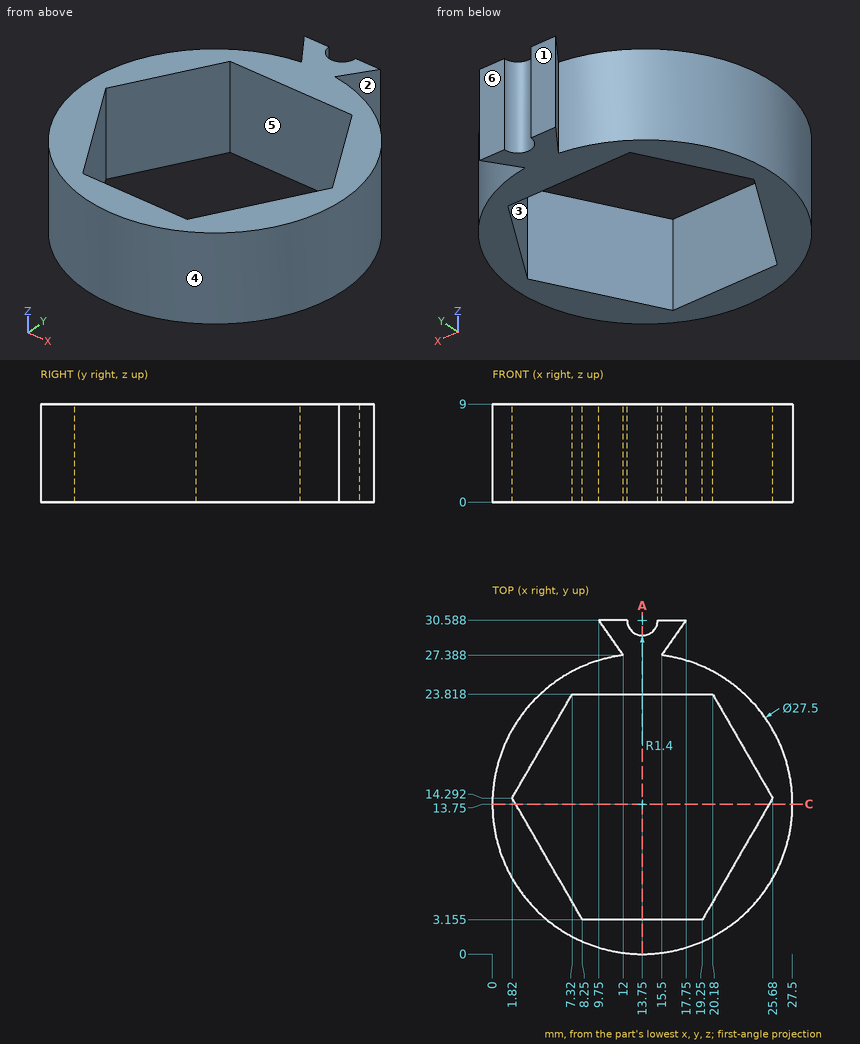
Source: three-view drawing plus pictorial views. Frame: mm from the lowest corner of the part. A direction names the side the tool comes from. Round coordinates to 2 decimals unless told otherwise and drop trailing zeros. Loops run counter-clockwise (first coordinate to the right, second up) from the corner with the lowest first, then second, coordinate; pieces in that order, holes last. Notation, with made-up numbers: (19, 38.5) - (63, 38.5) arc R27 ccw to (63, 57.5) - close; hole circle Ø6 at (45, -32.75). An arc over 180 degrees is marked (long way). Write item = value, one per line. Start each with the question number.
Item 1: First-contact query: pin 1 Ø1 at (x, z) = (11.5, 3.5) entering from -Y; pin 2 Ø5 at (y, z) = (21.5, 2) entering from -X; pin 3 Ø1 at (x, z) = (19, 3) entering from +Y; pin 4 Ø1.5 at (x, y) = (6, 9) entering from -Z. Flat tips, straight axial feed; report the tip coordinate or a pass-through.
Item 2: Section query C-C on y = 13.75. Output: boundary loops of the cut face in (x, z), plus the area to 3 significant figures.
Item 3: Reachability of the marked faces 1, 2 and 3 from +Z, -Z, +X, -X, +Y, -Y: full face, straight path, thin tool, end or side. Return the list, or none.
Item 4: Mould query, pull axis X, two halves, no side actions, for the marked faces 4, 5 and 6. Classes: released by +X, released by -X, zero draft, split by the parting line, or undercut.
Item 5: Material intervals for line 1 (Y direction, x = 16, z = 6.5) (1 decimal); line 2 (X direction, y = 17, z = 6.5); line 3 (X direction, y = 22.5, z = 7.5), sorted ascending.
Item 6: Section query A-A on x = 13.75. Output: boundary loops of the cut face in (y, z) (1 decimal), plus the area to 3 significant figures.
Results list:
q1.pin_1 = 0.11
q1.pin_2 = 1.04
q1.pin_3 = 26.65
q1.pin_4 = through
q2.outline = (0, 0) - (2.13, 0) - (2.13, 9) - (0, 9) - close; (25.37, 0) - (27.5, 0) - (27.5, 9) - (25.37, 9) - close
q2.area = 38.4 mm²
q3.face_1 = +Z, -Z, +X, -X, +Y
q3.face_2 = +Z, -Z, +X
q3.face_3 = +Z, -Z
q4.face_4 = split by the parting line
q4.face_5 = undercut
q4.face_6 = zero draft
q5.line_1 = 0.2 to 3.2, 23.8 to 27.3, 28.1 to 30.6
q5.line_2 = 0.39 to 3.38, 24.12 to 27.11
q5.line_3 = 3.14 to 6.56, 20.94 to 24.36
q6.outline = (0, 0) - (3.2, 0) - (3.2, 9) - (0, 9) - close; (23.8, 0) - (29.2, 0) - (29.2, 9) - (23.8, 9) - close
q6.area = 76.7 mm²
